Drawing for the job (mm, zero at the part's lowest x, y, z). A direction names the side the tool comes from. Give positions to 0.01 mm unless a question says otherwise; leave off trailing zeros. Order: outer loops, then holes, each group sorted by start corner. A loop starts at its lowest first (then second) coordinate and runs counter-clockwise, first axis right, second up. Notation, with made-up numbers: (22.25, 61) - (50.25, 61) arc R19 ccw to (50.25, 85) - close; hole circle Ø7 at (-32.5, -6). An arc over 180 degrees is marked (long way). Use a Markdown table: item, result. Add a question column.
(1) Slice it at C-C (y = 4.5). Write the cut outline in (x, z), then the cut area to 3 significant figures.
(2) Slice it at D-D (z = 20.5). Write the cut outline in (x, y).
(3) Slice it at A-A (x = 52). Write the cut outline in (y, z), then the cut area to 3 significant figures.
(4) Which spindle directions (+Z, -Z, +X, -X, +Y, -Y) get a long thin tool onto all of the face, cutting with end or side? Do the marked faces 3 and 4. Say none if no direction does.
(5) Mould opens along Z. For the marked faces 1 and 2 say: +Z half, -Z half, draft (parallel to the pull), parting line (faces both ways), or undercut.
(6) Slice it at B-B (z = 52). Write the cut outline in (x, y).
(7) Wall check: line 1 (Z direction, x = 52, y = 23); line 2 (Y direction, x = 63.5, z = 11); line 3 (X direction, y = 32, z = 53). Give the ranges that are in metal, low to high.
(8) Flat gauge pins, fed straight in: pin 1 (6 mm diameter, centred on x = 36, y = 11.5, fed in from +Z); pin 2 (3 mm diameter, centred on y = 19.5, z = 18.5, fed in from -X); pin 3 (12 mm diameter, centred on y = 6.5, z = 54, fed in from -X); pin 4 (12 mm diameter, centred on x = 91.5, y = 15.5, fed in from -Z). Where does each tip first touch, or does it go through?
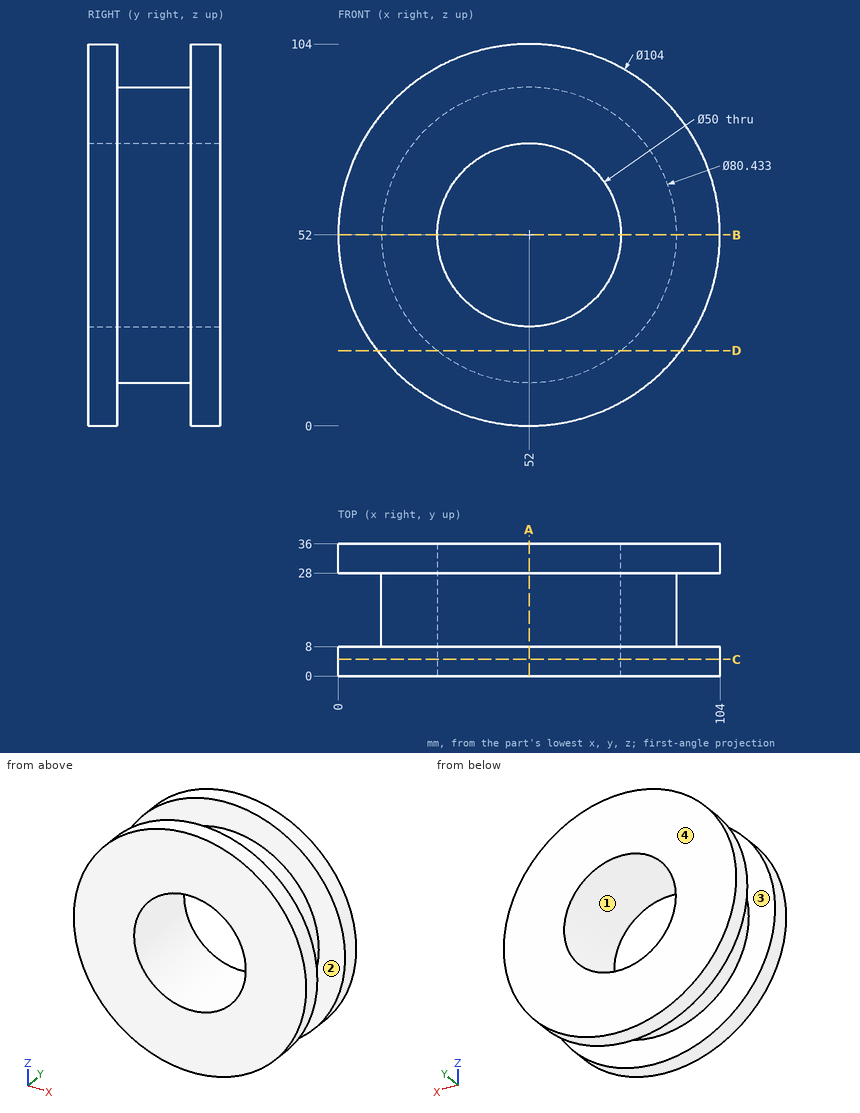
Solution:
| question | item | result |
|---|---|---|
| 1 | outline | circle Ø104 at (52, 52); hole circle Ø50 at (52, 52) |
| 1 | area | 6,530 mm2 |
| 2 | outline | (10.63, 0) - (93.37, 0) - (93.37, 8) - (77, 8) - (77, 28) - (93.37, 28) - (93.37, 36) - (10.63, 36) - (10.63, 28) - (27, 28) - (27, 8) - (10.63, 8) - close |
| 3 | outline | (0, 0) - (8, 0) - (8, 11.78) - (28, 11.78) - (28, 0) - (36, 0) - (36, 27) - (0, 27) - close; (0, 77) - (36, 77) - (36, 104) - (28, 104) - (28, 92.22) - (8, 92.22) - (8, 104) - (0, 104) - close |
| 3 | area | 1,470 mm2 |
| 4 | face 3 | none |
| 4 | face 4 | +Z, -Z, +X, -X, +Y |
| 5 | face 1 | undercut |
| 5 | face 2 | draft |
| 6 | outline | (0, 0) - (27, 0) - (27, 36) - (0, 36) - (0, 28) - (11.78, 28) - (11.78, 8) - (0, 8) - close; (77, 0) - (104, 0) - (104, 8) - (92.22, 8) - (92.22, 28) - (104, 28) - (104, 36) - (77, 36) - close |
| 7 | line 1 | 11.78 to 27, 77 to 92.22 |
| 7 | line 2 | 0 to 8, 28 to 36 |
| 7 | line 3 | 0.01 to 27.02, 76.98 to 103.99 |
| 8 | pin 1 | z = 90.06 |
| 8 | pin 2 | x = 27.64 |
| 8 | pin 3 | x = 0 |
| 8 | pin 4 | z = 29.75 |
